Source: three-view drawing plus pictorial views. Frame: mm from the lowest corner of the part. A direction names the side the tool comes from. Round coordinates to 2 decimals unless told otherwise and drop trailing zeros. Loops run counter-clockwise (first coordinate to the right, second up) from the corner with the lowest first, then second, coordinate; pieces in that order, holes last. Notation, with made-up numbers: M 6,3 L 48,3 A31 cw 48,30 Z; hole C 60.5,84 d9. An arc over 180 degrees is marked long. Write each question's results on one line, items separated by ' | '.
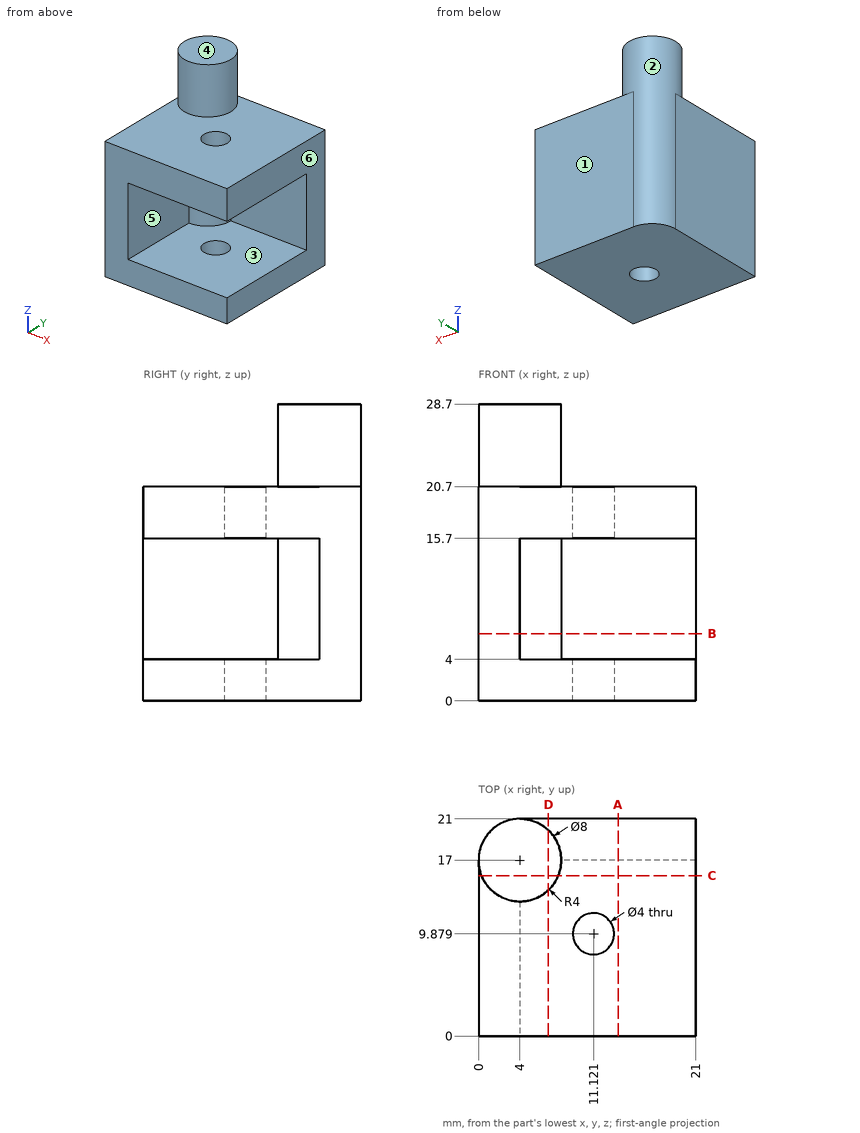
1. Draft query along Z for the marked faces 4, 5 and 6. Return one class per face: pulls with the +Z half, pulls with the -Z half, needs draft (parallel to the pull), parting line crosses it, or undercut.
Answer key:
face 4: pulls with the +Z half | face 5: undercut | face 6: needs draft
2. Pin query (flat end, axial travel): P1, Ø1.5, axis at x = 14.5, z = 7, coming from the -Y side; P2, Ø5, axis at x = 12.5, y = 7.5, coming from the +Z side; P3, Ø3, axis at x = 11.12, y = 9.88, coming from the -Z side; P4, Ø3, axis at x = 8, z = 24.5, coming from the -Y side. Return the tip coordinate at first contact, or that it passes through.
Answer key:
P1: stops at y = 17 | P2: stops at z = 20.7 | P3: passes through | P4: stops at y = 13.88
3. Section C-C (y = 15.5). Output: boundary loops of the cut face in (x, z).
Answer key:
outline: M 0,0 L 21,0 L 21,4 L 7.71,4 L 7.71,15.7 L 21,15.7 L 21,20.7 L 7.71,20.7 L 7.71,28.7 L 0.29,28.7 L 0.29,20.7 L 0,20.7 Z
4. Section A-A (x = 13.5). Output: boundary loops of the cut face in (y, z).
Answer key:
outline: M 0,0 L 21,0 L 21,20.7 L 0,20.7 L 0,15.7 L 17,15.7 L 17,4 L 0,4 Z
5. Section D-D (x = 6.75). Output: boundary loops of the cut face in (y, z) (1 decimal), then the cut area to 3 significant figures.
Answer key:
outline: M 0,0 L 21,0 L 21,20.7 L 19.9,20.7 L 19.9,28.7 L 14.1,28.7 L 14.1,20.7 L 0,20.7 L 0,15.7 L 14.1,15.7 L 14.1,4 L 0,4 Z | area: 316 mm²
6. Section B-B (z = 6.5). Output: boundary loops of the cut face in (x, y).
Answer key:
outline: M 0,0 L 4,0 L 4,13 A4 ccw 8,17 L 21,17 L 21,21 L 4,21 A4 ccw 0,17 Z
7. Access query for the marked faces 1, 2 and 3. Directions: +Z, -Z, +X, -X, +Y, -Y. A direction counts if a zero-diameter tool reaches every point of the face in a straight line with its end or side. Return the directions, or none.
Answer key:
face 1: +Z, -Z, +X, -X, +Y | face 2: +Z | face 3: +X, -Y
8. Ray query, probe 1 along Z at (x, y) = (4.75, 5.5); probe 2 along X at (y, z) = (1.25, 6); probe 3 along Z at (x, y) = (16.75, 17.25). Return the intervals inside material, ascending.
Answer key:
probe 1: z = 0 to 4, 15.7 to 20.7 | probe 2: x = 0 to 4 | probe 3: z = 0 to 20.7
